Source: three-view drawing plus pictorial views. Frame: mm from the lowest corner of the part. Give positions to 0.01 mm unless a question says otherwise; leave off trailing zeros. Loops run counter-clockwise (first coordinate to the right, second up) from the corner with the lowest first, then second, coordinate; pieces in that order, holes last. Notation, with made-up numbers: M 47,57 L 83,57 A20 ccw 83,69 Z; hole C -21,78.5 d3. An arc over 180 degrees is marked long. One line per item, written item: value. Start each with the question number.
(1) Section B-B on x = 16.5. Output: boundary loops of the cut face in (y, z), plus the area to 3 significant figures.
(2) Pin query (flat end, axial travel): P1, Ø4, axis at x = 16.5, z = 43, coming from the +Y side; P2, Ø5, axis at x = 60, z = 6, coming from the -Y side (1 decimal); P3, Ø5, axis at y = 29, z = 11, coming from the -X side (1 decimal). Return the tip coordinate at first contact, or that it passes through.
(3) Ray query, line 1 along X through (y, z) = (22, 7) (1 decimal); line 2 along Y through (x, z) = (76, 19) (1 decimal); line 3 along Y through (x, z) = (25.5, 33) (1 decimal). Return the intervals inside material, ascending. Write a range as from..to.
(4) Section C-C on y = 29.5. Output: boundary loops of the cut face in (x, z) (1 decimal), plus the area to 3 significant figures.
(5) Pull-direction query (X, two-part tool) for the marked faces 1, 2 and 3; classes: released by +X, released by -X, zero draft, split by the parting line, or undercut.
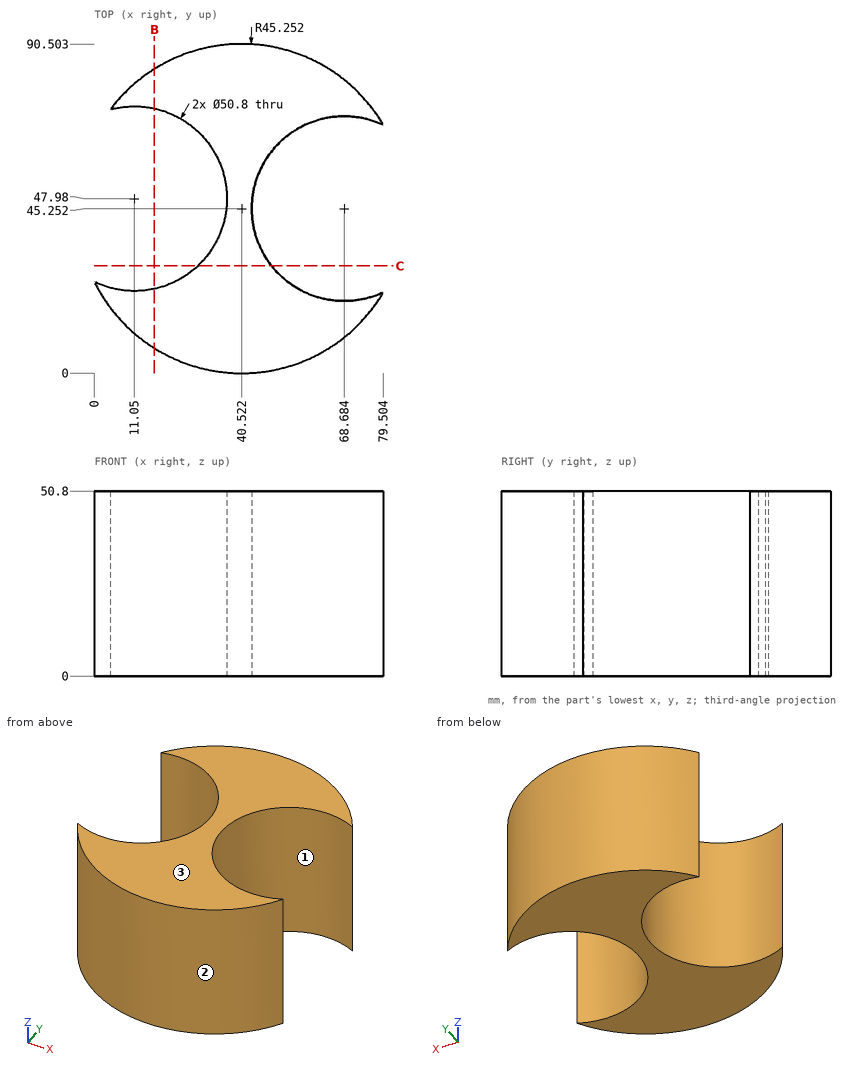
Output values:
1. outline: M 6.9,0 L 23.17,0 L 23.17,50.8 L 6.9,50.8 Z; M 72.79,0 L 83.6,0 L 83.6,50.8 L 72.79,50.8 Z
1. area: 1,380 mm²
2. P1: stops at y = 84.78
2. P2: stops at y = 3.3
2. P3: stops at x = 24.6
3. line 1: x = 1.7..58.5, 78.9..79.3
3. line 2: y = 17.2..20.9, 69.6..73.3
3. line 3: y = 2.6..27.1, 68.9..87.9
4. outline: M 28.5,0 L 48.8,0 L 48.8,50.8 L 28.5,50.8 Z
4. area: 1,030 mm²
5. face 1: undercut
5. face 2: split by the parting line
5. face 3: zero draft
